Check sheet for the modelled part. Datum: model origin and axes. Units: mm. Give positions to 0.01 mm unless a question says otherwise; leave off trailing zeros. Write each loop counter-clockwise with the first axis right and the second up, starting at its lowest first coordinate (ties: lowest second). Pieces come first, ordered by that corner, then holes. Notation, with made-up numbers: M -25.5,5.5 L -7.5,5.5 A4 cw -7.5,10.5 Z; hole C 77,51.25 d2. An arc over 180 degrees is marked long. Write each question's results on one line, items separated by ' | '. Start each with the question number.
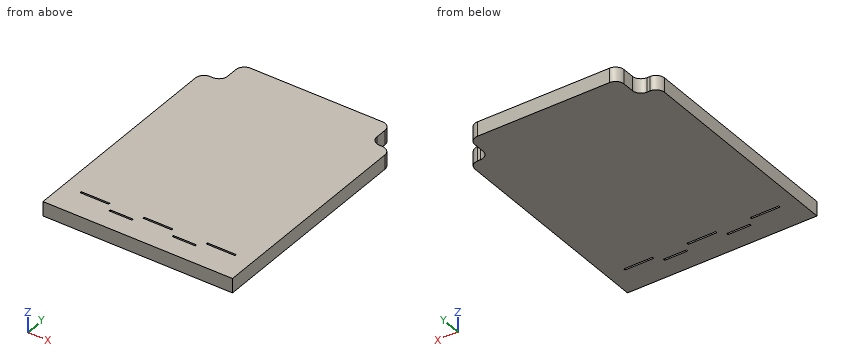
from build123d import *

# Parameters (mm, degrees)
F0_W     = 330
F0_H     = 390
F1_DEPTH = 25
F2_W     = 260
F2_H     = 25
F3_DEPTH = 50
F4_R     = 15
F5_W     = 50
F5_H     = 3
F5_W_2   = 40
F6_DEPTH = 25


with BuildPart() as f1:
    # F0 (on Top) → F1 (new body)
    with BuildSketch(Plane.XY):
        Rectangle(F0_W, F0_H)
    extrude(amount=F1_DEPTH)

    # F2 (on face) → F3 (join)
    with BuildSketch(Plane(origin=(0, 195, 0), x_dir=(-1, 0, 0), z_dir=(0, 1, 0))):
        with Locations((0, 12.5)):
            Rectangle(F2_W, F2_H)
    extrude(amount=F3_DEPTH)

    # F4
    f4_edges = [f1.edges().sort_by_distance(p)[0] for p in [
        (-165, 195, 12.5),
        (-130, 245, 12.5),
        (130, 245, 12.5),
        (165, 195, 12.5),
        (-130, 195, 12.5),
        (130, 195, 12.5),
    ]]
    fillet(f4_edges, radius=F4_R)

    # F5 (on face) → F6 (cut)
    with BuildSketch(Plane.XY.offset(25)):
        with Locations((-110, -145.050164)):
            Rectangle(F5_W, F5_H)
        with Locations((0, -145.050164)):
            Rectangle(F5_W, F5_H)
        with Locations((110, -145.050164)):
            Rectangle(F5_W, F5_H)
        with Locations((-55, -158.050164)):
            Rectangle(F5_W_2, F5_H)
        with Locations((55, -158.050164)):
            Rectangle(F5_W_2, F5_H)
    extrude(amount=-F6_DEPTH, mode=Mode.SUBTRACT)


solid = f1.part
Q1. Scan lines: L1, parallel to X at y = -159.5, z = 4.5; L2, parallel to Y at x = 57.5, z = 5; L3, parallel to Y at x = 11.5, z = 23.25. Record each from-to range of solid material in increasing order.
Q2. Section check B-B on y = 189.5. Record the boundary of the cut face in (x, z).
Q3. Depth check by flat-ended pin: pin 1 Ø5.5 at (x, z) = (148.5, 10) entering from +Y; pin 2 Ø10 at (x, z) = (-122.5, 7.5) entering from +Y. Enter the tip coordinate at first touch or a pass-through.
Q4. Section check A-A on z = 16.25. State how many separate pieces and enclosed holes the cut face has, plus the area to 3 significant figures.
Check result:
1) L1: -165 to -75, -35 to 35, 75 to 165 | L2: -195 to -159.55, -156.55 to 245 | L3: -195 to -146.55, -143.55 to 245
2) outline: M -161.61,0 L 161.61,0 L 161.61,25 L -161.61,25 Z
3) pin 1: y = 195 | pin 2: y = 244.79
4) separate pieces: 1 | enclosed holes: 5 | area: 141,000 mm^2
